Answer from the drawing. Dimensions are ordinates in mm from the lowest x, y and z of the part. A direction names the side the tool comes from. Round coordinates to 2 decimals unless told otherwise and drop trailing zeros. Order: outer loops, then holes, each group sorted by start corner. A loop starts at its lowest first (then second) coordinate and runs counter-clockwise, first axis right, second up. Notation, with made-up numbers: (12, 19) -> (51, 19) arc R21 cw to (51, 48) -> close; hole circle Ø10 at (0, 20.25). An arc over 180 degrees is marked (long way). Use a Markdown table: item, result. Add a question column.
1. Section C-C, the plane y = 4.1 is taken. Give the vertices of the cut face in (x, z).
2. Section D-D, the plane z = 15 is taken. Give the vertices of the cut face in (x, y).
3. Section A-A, the plane z = 24 is taken. Give the vertices of the cut face in (x, y).
4. Given pin 1 (5 mm diameter, centred on x = 15, z = 24, fed in from +Y); pin 2 (3 mm diameter, centred on x = 6, z = 15, fed in from +Y); pin 3 (2 mm diameter, centred on y = 1, z = 16.5, fed in from -X); pin 4 (1 mm diameter, centred on x = 11, y = 4, fed in from -Z), each flat-ended and moving along its own axis, determine where each tip first touches the part or whether it passes through.
5. Section B-B, the plane x = 15 is taken. Give the vertices of the cut face in (y, z).
6. For the marked faces 1 and 2, determine the directions among +Z, -Z, +X, -X, +Y, -Y from which every point of the face is accessible in a straight line to the end or side of a thin tool.
7. Consider L1, parallel to X at y = 4.05, z = 15; L2, parallel to X at y = 1.2, z = 15; L3, parallel to Z at x = 16.75, y = 3.7. Determine where each line is inside the solid, lowest interval first. Write a range as [from, to].
8. The mould has two halves that part along X. Classify the marked faces 3, 4, 5 and 6: +X half, -X half, draft (parallel to the pull), parting line (faces both ways), or undercut.
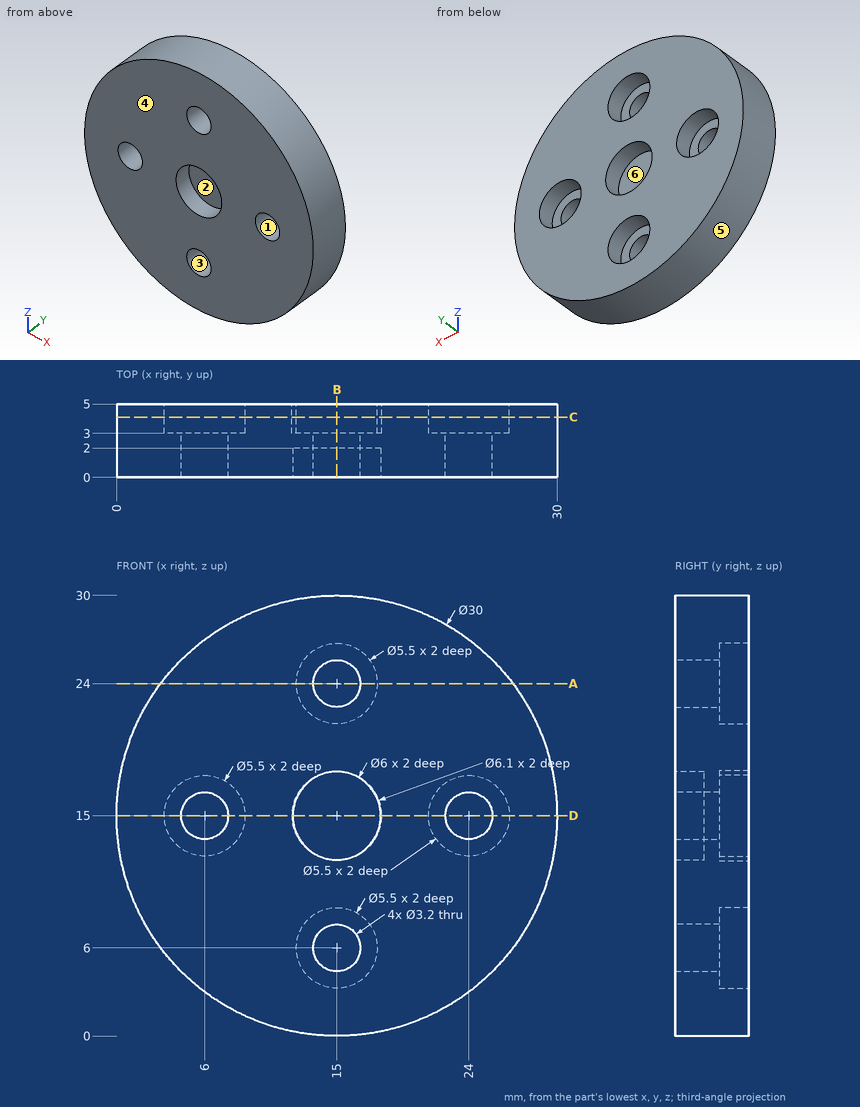
Verdict:
| question | item | result |
|---|---|---|
| 1 | outline | circle Ø30 at (15, 15); hole circle Ø5.5 at (6, 15); hole circle Ø6.1 at (15, 15); hole circle Ø5.5 at (15, 6); hole circle Ø5.5 at (15, 24); hole circle Ø5.5 at (24, 15) |
| 2 | outline | (0, 0) -> (4.4, 0) -> (4.4, 3) -> (3.25, 3) -> (3.25, 5) -> (0, 5) -> close; (7.6, 0) -> (12, 0) -> (12, 2) -> (18, 2) -> (18, 0) -> (22.4, 0) -> (22.4, 3) -> (21.25, 3) -> (21.25, 5) -> (18.05, 5) -> (18.05, 3) -> (11.95, 3) -> (11.95, 5) -> (8.75, 5) -> (8.75, 3) -> (7.6, 3) -> close; (25.6, 0) -> (30, 0) -> (30, 5) -> (26.75, 5) -> (26.75, 3) -> (25.6, 3) -> close |
| 3 | outline | (3, 0) -> (13.4, 0) -> (13.4, 3) -> (12.25, 3) -> (12.25, 5) -> (3, 5) -> close; (16.6, 0) -> (27, 0) -> (27, 5) -> (17.75, 5) -> (17.75, 3) -> (16.6, 3) -> close |
| 4 | pin 1 | stops at y = 3 |
| 4 | pin 2 | passes through |
| 4 | pin 3 | stops at x = 0.01 |
| 4 | pin 4 | stops at z = 0.41 |
| 5 | outline | (0, 0) -> (5, 0) -> (5, 3.25) -> (3, 3.25) -> (3, 4.4) -> (0, 4.4) -> close; (0, 7.6) -> (3, 7.6) -> (3, 8.75) -> (5, 8.75) -> (5, 11.95) -> (3, 11.95) -> (3, 18.05) -> (5, 18.05) -> (5, 21.25) -> (3, 21.25) -> (3, 22.4) -> (0, 22.4) -> (0, 18) -> (2, 18) -> (2, 12) -> (0, 12) -> close; (0, 25.6) -> (3, 25.6) -> (3, 26.75) -> (5, 26.75) -> (5, 30) -> (0, 30) -> close |
| 6 | face 1 | +Y, -Y |
| 6 | face 2 | -Y |
| 7 | L1 | x = [0, 3.25], [8.75, 11.95], [18.05, 21.25], [26.75, 30] |
| 7 | L2 | x = [0, 4.4], [7.6, 12], [18, 22.4], [25.6, 30] |
| 7 | L3 | z = [0.1, 3.88], [8.12, 12.5], [17.5, 21.88], [26.12, 29.9] |
| 8 | face 3 | undercut |
| 8 | face 4 | draft |
| 8 | face 5 | parting line |
| 8 | face 6 | undercut |
